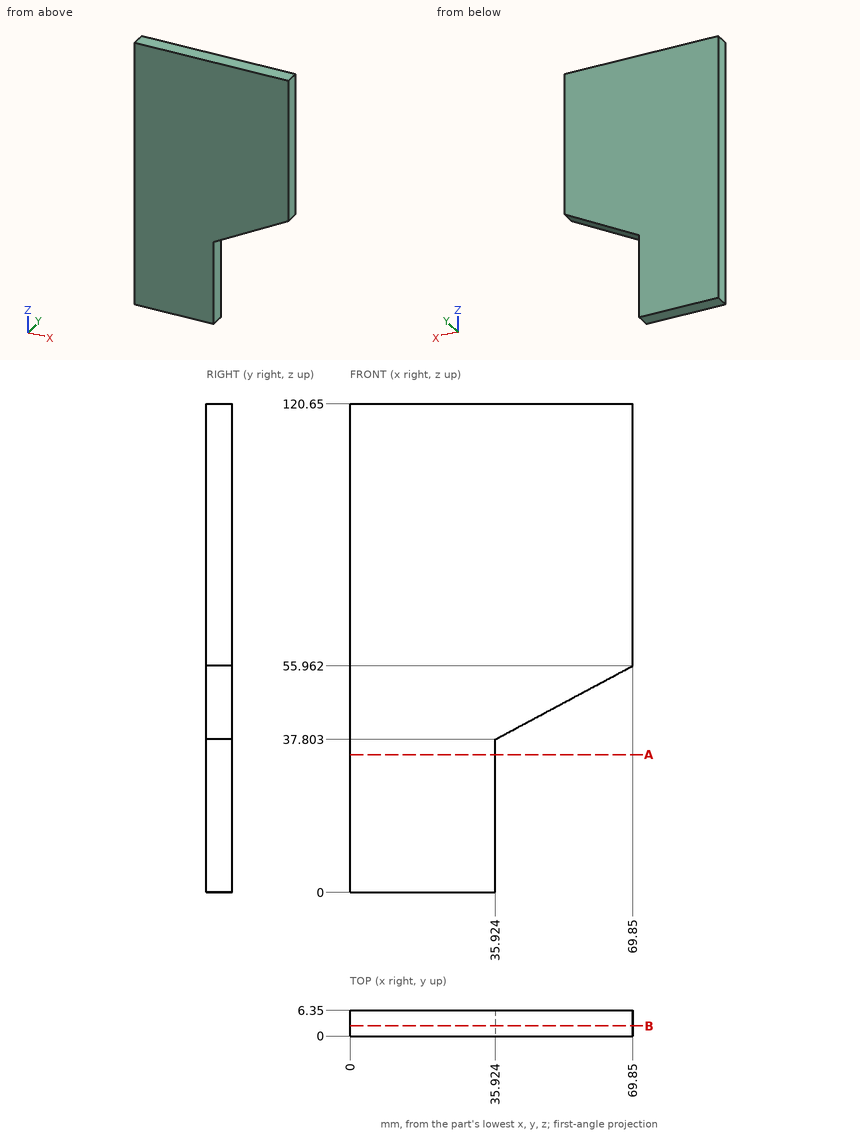
Geometry: see drawing. Coordinates: mm, zero at the bounding-box minimum. Coordinates: 2 decimals unless noted, no trailing zeros. Write each loop counter-clockwise with the first axis right and the second up, starting at its lowest first coordinate (ties: lowest second). Pieces come first, ordered by that corner, then holes. Notation, with made-up numbers: (80, 56.5) - (135, 56.5) arc R20 ccw to (135, 65.5) - close; hole circle Ø10 at (25.25, -0.5). An arc over 180 degrees is marked (long way). Put each result on its own line as item: value. Start each with the question number.
1) Cut plane B-B (y = 2.5). Return the cut outline in (x, z).
2) Ray query, L1, parallel to X at y = 1.5, z = 10.5; L2, parallel to X at y = 1, z = 45.5 (1 decimal); L3, parallel to Z at x = 52, y = 0.5. Return the intervals inside material, ascending.
3) Cut plane A-A (z = 34). Return the cut outline in (x, y), plus the area to 3 significant figures.
4) Contact query for flat-ended pins moving along their axis: pin 1 (1 mm diameter, centred on x = 60.5, y = 2.5, fed in from -Z); pin 2 (3 mm diameter, centred on y = 1, z = 21.5, fed in from +X); pin 3 (1.5 mm diameter, centred on x = 23.5, z = 85, fed in from -Y). Output: stop coordinate, or through.
Resolved:
1. outline: (0, 0) - (35.92, 0) - (35.92, 37.8) - (69.85, 55.96) - (69.85, 120.65) - (0, 120.65) - close
2. L1: x = 0 to 35.92
2. L2: x = 0 to 50.3
2. L3: z = 46.41 to 120.65
3. outline: (0, 0) - (35.92, 0) - (35.92, 6.35) - (0, 6.35) - close
3. area: 228 mm2
4. pin 1: stops at z = 50.69
4. pin 2: stops at x = 35.92
4. pin 3: stops at y = 0
